```python
from build123d import *

# Parameters (mm, degrees)
F0_W     = 60
F0_H     = 25
F1_DEPTH = 10
F2_W     = 6
F2_H     = 25
F3_DEPTH = 3
F6_D     = 6.3
F7_DEPTH = 5


with BuildPart() as f1:
    # F0 (on Top) → F1 (new body)
    with BuildSketch(Plane.XY):
        with Locations((30, 12.5)):
            Rectangle(F0_W, F0_H)
    extrude(amount=F1_DEPTH)

    # F2 (on face) → F3 (cut)
    with BuildSketch(Plane.XY.offset(10)):
        with Locations((6, 12.5)):
            Rectangle(F2_W, F2_H)
        with Locations((42, 12.5)):
            Rectangle(F2_W, F2_H)
    extrude(amount=-F3_DEPTH, mode=Mode.SUBTRACT)

    # F6 (through all)
    with Locations(Plane(origin=(0, 0, 0), x_dir=(1, 0, 0), z_dir=(0, 0, -1))):
        with Locations((15, -12.5), (52, -12.5)):
            Hole(F6_D / 2)

    # F5 (on face) → F7 (cut)
    with BuildSketch(Plane(origin=(0, 0, 0), x_dir=(1, 0, 0), z_dir=(0, 0, -1))):
        Polygon((21.119913, -12.5), (18.059956, -7.2), (11.940044, -7.2), (8.880087, -12.5), (11.940044, -17.8), (18.059956, -17.8), align=None)
        Polygon((45.880087, -12.5), (48.940044, -17.8), (55.059956, -17.8), (58.119913, -12.5), (55.059956, -7.2), (48.940044, -7.2), align=None)
    extrude(amount=-F7_DEPTH, mode=Mode.SUBTRACT)


solid = f1.part
```
Input: part model. Units: mm. Frame: model coordinates. A direction names the side the tool comes from. Give positions to 0.01 mm unless a question says otherwise; leave off trailing zeros. Loops run counter-clockwise (first coordinate to the right, second up) from the corner with the lowest first, then second, coordinate; pieces in that order, holes last. Notation, with made-up numbers: M 28.25,76 L 76.25,76 A16 cw 76.25,105 Z; hole C 15,31.25 d3. An arc over 180 degrees is marked long. Answer as CSV lines item,"result". Start each with the question number.
1. Section B-B on x = 52. Return loops of the section in (y, z).
2. Line query: L1, parallel to X at y = 7, z = 8.75; L2, parallel to X at y = 12.5, z = 7.8; L3, parallel to X at y = 12.5, z = 6.75. Output: solid intervals per line, ascending.
3. Pull-direction query (Y, two-part tool) for faces 4 (the face through (15, 7.2, 2)), 5 (the face through (19.569, 15.187, 2.465)), 6 (the face through (30, 0, 5)), 7 (the face through (9, 12, 9)); classes: released by +Y, released by -Y, zero draft, split by the parting line, or undercut.
4. Pin query (flat end, axial travel): P1, Ø4, axis at x = 42, y = 13, coming from the +Z side; P2, Ø4, axis at x = 15, y = 12.5, coming from the -Z side (1 decimal). Return the tip coordinate at first contact, or that it passes through.
5. Section C-C on y = 13.75. Return loops of the section in (x, z), plus the area to 3 significant figures.
6. Reachability of faces 1 (the face through (54.1, 15.5, 10)), 2 (the face through (3, 12, 9)), 3 (the face through (18, 10, 5)) from +Z, -Z, +X, -X, +Y, -Y: full face, straight path, thin tool, end or side. Return the list, or none.
7. Section A-A on z = 1. Return loops of the section in (x, y), plus the area to 3 significant figures.
Computed values:
1,outline,"M 0,0 L 7.2,0 L 7.2,5 L 9.35,5 L 9.35,10 L 0,10 Z; M 15.65,5 L 17.8,5 L 17.8,0 L 25,0 L 25,10 L 15.65,10 Z"
2,L1,"x = 0 to 3, 9 to 39, 45 to 60"
2,L2,"x = 0 to 3, 9 to 11.85, 18.15 to 39, 45 to 48.85, 55.15 to 60"
2,L3,"x = 0 to 11.85, 18.15 to 48.85, 55.15 to 60"
3,face 4,"undercut"
3,face 5,"undercut"
3,face 6,"released by -Y"
3,face 7,"zero draft"
4,P1,"stops at z = 7"
4,P2,"passes through"
5,outline,"M 0,0 L 9.6,0 L 9.6,5 L 12.11,5 L 12.11,10 L 9,10 L 9,7 L 3,7 L 3,10 L 0,10 Z; M 17.89,5 L 20.4,5 L 20.4,0 L 46.6,0 L 46.6,5 L 49.11,5 L 49.11,10 L 45,10 L 45,7 L 39,7 L 39,10 L 17.89,10 Z; M 54.89,5 L 57.4,5 L 57.4,0 L 60,0 L 60,10 L 54.89,10 Z"
5,area,"398 mm²"
6,face 1,"+Z, +X, -X, +Y, -Y"
6,face 2,"+Z, +Y, -Y"
6,face 3,"-Z"
7,outline,"M 0,0 L 60,0 L 60,25 L 0,25 Z; hole M 8.88,12.5 L 11.94,7.2 L 18.06,7.2 L 21.12,12.5 L 18.06,17.8 L 11.94,17.8 Z; hole M 45.88,12.5 L 48.94,7.2 L 55.06,7.2 L 58.12,12.5 L 55.06,17.8 L 48.94,17.8 Z"
7,area,"1,310 mm²"
